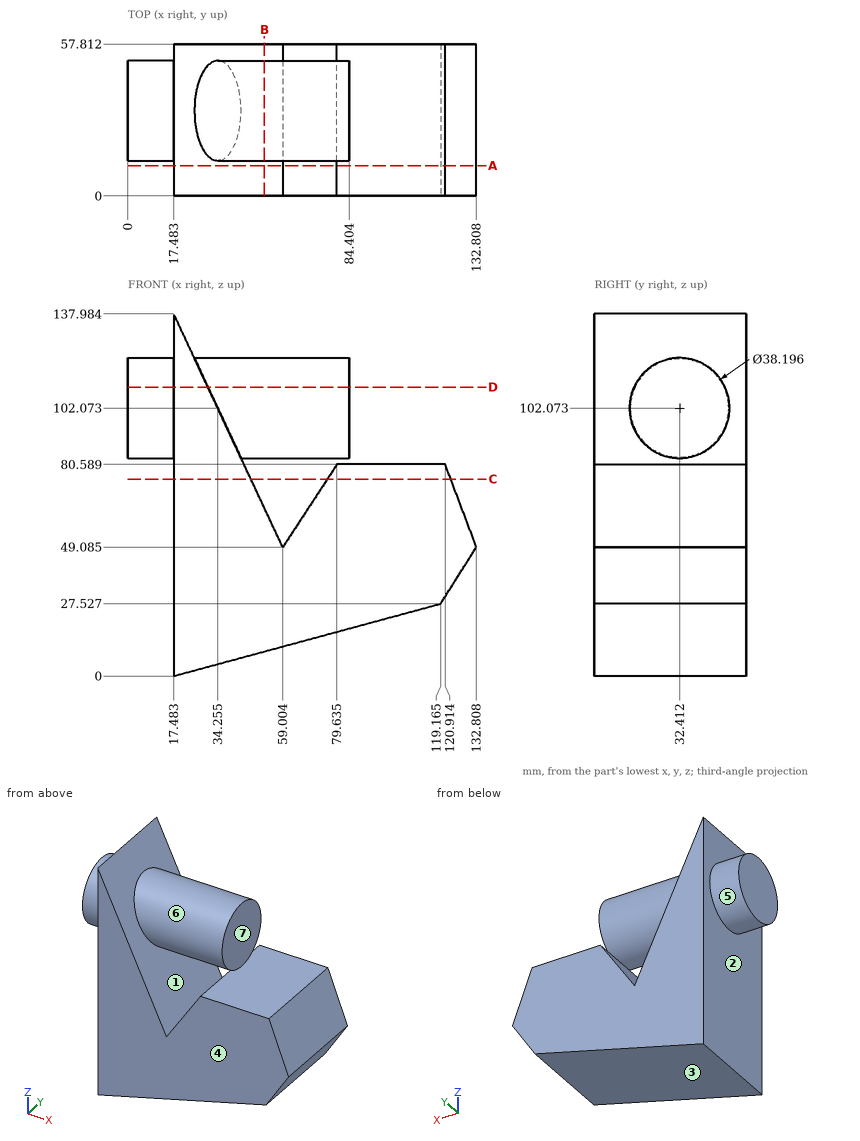
Part print with two shaded views. Sizes in mm from the minimum x, y, z corner. A direction names the side the tool comes from. Round coordinates to 2 decimals unless told otherwise and drop trailing zeros. Loops run counter-clockwise (first coordinate to the right, second up) from the corner with the lowest first, then second, coordinate; pieces in that order, holes last.
Item 1: Saw through at C-C (z = 75). List the corners of the cut face in (x, y) (1 decimal), then the cut area to 3 significant figures.
Item 2: Pin check, flat tips, straight feed: P1, Ø2, axis at x = 67, z = 98, coming from the -Y side; P2, Ø4, axis at x = 47.5, y = 34.5, coming from the -Z side (1 decimal); P3, Ø3, axis at y = 28, z = 45.5, coming from the -X side; P4, Ø10, axis at x = 104.5, z = 16.5, coming from the -Y side. Stop position of each tip, or through.
Item 3: Saw through at D-D (z = 110). List the corners of the cut face in (x, y), then the cut area to 3 significant figures.
Item 4: Drill centre lines: line 1 along X through (y, z) = (48, 101); line 2 along X through (y, z) = (28, 65) (1 decimal); line 3 along Z through (x, y) = (53, 25.5) (1 decimal). Where is each one in solid material? Low to high.
Item 5: Two-plate mould, pull along X, no slides. Class the marked faces 1, 2 and 3: released by +X, released by -X, zero draft, split by the parting line, or undercut.
Item 6: Which spindle directions (+Z, -Z, +X, -X, +Y, -Y) get a long thin tool onto all of the face, cutting with end or side? Do the marked faces 4, 5, 6 and 7. Say none if no direction does.
Item 7: Saw through at A-A (y = 11.5). List the corners of the cut face in (x, z) (1 decimal), then the cut area to 3 significant figures.
Item 8: Saw through at B-B (x = 52). List the corners of the cut face in (y, z) (1 decimal), then the cut area to 3 significant figures.
Worked answers:
1. outline: (17.5, 0) - (46.9, 0) - (46.9, 57.8) - (17.5, 57.8) - close; (76, 0) - (123, 0) - (123, 57.8) - (76, 57.8) - close
1. area: 4,420 mm2
2. P1: stops at y = 13.56
2. P2: stops at z = 7.6
2. P3: stops at x = 17.48
2. P4: passes through
3. outline: (0, 15.04) - (17.48, 15.04) - (17.48, 0) - (30.55, 0) - (30.55, 15.04) - (84.4, 15.04) - (84.4, 49.79) - (30.55, 49.79) - (30.55, 57.81) - (17.48, 57.81) - (17.48, 49.79) - (0, 49.79) - close
3. area: 3,230 mm2
4. line 1: x = 0 to 84.4
4. line 2: x = 17.5 to 51.6, 69.4 to 126.8
4. line 3: z = 9.6 to 61.9, 84.3 to 119.9
5. face 1: undercut
5. face 2: released by -X
5. face 3: released by +X
6. face 4: +Z, -Z, +X, -X, -Y
6. face 5: -X
6. face 6: +X
6. face 7: +Z, +X, +Y, -Y
7. outline: (17.5, 0) - (119.2, 27.5) - (132.8, 49.1) - (120.9, 80.6) - (79.6, 80.6) - (59, 49.1) - (17.5, 138) - close
7. area: 7,400 mm2
8. outline: (0, 9.3) - (57.8, 9.3) - (57.8, 64.1) - (0, 64.1) - close; circle Ø38.2 at (32.4, 102.1)
8. area: 4,310 mm2
